```python
from build123d import *

# Parameters (mm, degrees)
SKETCH1_W           = 24
SKETCH1_H           = 22.5
BOSS_EXTRUDE1_DEPTH = 1.6
SKETCH2_W           = 6.4
SKETCH2_H           = 6.4
BOSS_EXTRUDE2_DEPTH = 1.5
SKETCH3_R           = 2.65
BOSS_EXTRUDE3_DEPTH = 7.9
SKETCH4_R           = 0.45
CUT_EXTRUDE1_DEPTH  = 3.6
LPATTERN1_COUNT     = 8
LPATTERN1_PITCH     = 2.54


with BuildPart() as part:
    # Sketch1 → Boss-Extrude1 (new body)
    with BuildSketch(Plane(origin=(0, 0, 0), x_dir=(1, 0, 0), z_dir=(0, 1, 0))):
        Rectangle(SKETCH1_W, SKETCH1_H)
    extrude(amount=BOSS_EXTRUDE1_DEPTH)

    # Sketch2 → Boss-Extrude2 (add)
    with BuildSketch(Plane(origin=(12, 0, 0), x_dir=(0, 0, -1), z_dir=(1, 0, 0))):
        with Locations((0.431041527, 2.2)):
            Rectangle(SKETCH2_W, SKETCH2_H)
    extrude(amount=BOSS_EXTRUDE2_DEPTH)

    # Sketch3 → Boss-Extrude3 (add)
    with BuildSketch(Plane(origin=(13.5, 0, 0), x_dir=(0, 0, -1), z_dir=(1, 0, 0))):
        with Locations((0.431041527, 2.2)):
            Circle(SKETCH3_R)
    extrude(amount=BOSS_EXTRUDE3_DEPTH)

    # Sketch4 → Cut-Extrude1 (cut, through all)
    with BuildSketch(Plane(origin=(0, 1.6, 0), x_dir=(1, 0, 0), z_dir=(0, 1, 0))):
        with Locations((-10.5, -9.15)):
            Circle(SKETCH4_R)
    cut_extrude1 = extrude(amount=-CUT_EXTRUDE1_DEPTH, mode=Mode.SUBTRACT)

    # LPattern1: Cut-Extrude1 ×8
    with Locations(*[(0, 0, -i * LPATTERN1_PITCH) for i in range(1, LPATTERN1_COUNT)]):
        add(cut_extrude1, mode=Mode.SUBTRACT)


solid = part.part
```
Design review of the part built by this model. Coordinates are the model's own, in mm. A direction names the side the tool comes from. Coordinates: 2 decimals unless noted, no trailing zeros. Order: outer loops, then holes, each group sorted by start corner. A loop starts at its lowest first (then second) coordinate and runs counter-clockwise, first axis right, second up.
1) For faces 5 (the flat face through (0, 0, 0)), 6 (the flat face through (0, 1.6, 0)), 7 (the cylindrical face through (-10.071, 0.811, -1.145)), 8 (the cylindrical face through (17.395, 0.588, 1.672)), list the 3-axis set-ups (+Z, -Z, +X, -X, +Y, -Y) from which the entire face can be reached by the end or side of a thin tool; tool diameter is ignored.
2) Mouldability with a two-part tool opening along X and no side actions: class faces 1 (the flat face through (12, 1, 7)), 2 (the cylindrical face through (-10.29, 0.81, 1.93)), 3 (the flat face through (12, 4, 0)), 4 (the flat face through (13, 2, 2.769)) as +X half, -X half, draft (parallel to the pull), parting line (faces both ways), or undercut.
3) Wall thickness on line 1 along X through (y, z) = (1.35, 4.07); line 2 along Y through (x, z) = (-1, 9.5); line 3 along X through (y, z) = (-0.25, 1.25): over which ranges is each line inside the solid? List them lowest first.
4) Take a section at D-D, the plane z = -1.01. Give the boundary of the cut face in (x, y).
5) Take a section at B-B, the plane y = 1.25. State how many separate pieces and enclosed holes the cut face has, and give its area (3 significant figures).
6) Clearance check with flat-ended pins moving along their axes: pin 1 (6 mm diameter, centred on x = 17, z = -1.5, fed in from +Y); pin 2 (1.9 mm diameter, centred on y = 4.5, z = -1, fed in from -X); pin 3 (1.8 mm diameter, centred on y = 0.5, z = 7, fed in from +X). State where each tip first meets the part, or that it passes through.
7) Take a section at A-A, the plane z = 6.61. Give the boundary of the cut face in (x, y).
Returned:
1. face 5: +Z, -Z, -X, -Y
1. face 6: +Z, -Z, -X, +Y
1. face 7: +Y, -Y
1. face 8: +X
2. face 1: +X half
2. face 2: undercut
2. face 3: -X half
2. face 4: draft
3. line 1: x = -12 to -10.95, -10.05 to 12
3. line 2: y = 0 to 1.6
3. line 3: x = 12 to 13.5
4. outline: (-12, 0) - (-10.95, 0) - (-10.95, 1.6) - (-12, 1.6) - close; (-10.05, 0) - (12, 0) - (12, -1) - (13.5, -1) - (13.5, -0.39) - (21.4, -0.39) - (21.4, 4.79) - (13.5, 4.79) - (13.5, 5.4) - (12, 5.4) - (12, 1.6) - (-10.05, 1.6) - close
5. separate pieces: 1
5. enclosed holes: 8
5. area: 584 mm2
6. pin 1: stops at y = 4.85
6. pin 2: stops at x = 12
6. pin 3: stops at x = 12
7. outline: (-12, 0) - (-10.95, 0) - (-10.95, 1.6) - (-12, 1.6) - close; (-10.05, 0) - (12, 0) - (12, 1.6) - (-10.05, 1.6) - close
